```python
from build123d import *

# Parameters (mm, degrees)
SKETCH_1_R      = 12.5
EXTRUDE_1_DEPTH = 5
EXTRUDE_2_DEPTH = 5


with BuildPart() as part:
    # ｽｹｯﾁ1 → ﾎﾞｽ - 押し出し1 (new body)
    with BuildSketch(Plane.XY):
        with Locations((-14.880131723, 17.607142857)):
            Circle(SKETCH_1_R)
    extrude(amount=EXTRUDE_1_DEPTH)

    # ｽｹｯﾁ2 → ﾎﾞｽ - 押し出し2 (add)
    with BuildSketch(Plane(origin=(0, 0, 0), x_dir=(-1, 0, 0), z_dir=(0, 0, -1))):
        Polygon((13.880131723, 30.067078652), (16.678684785, 29.977074421), (18.364346975, 35.725860639), (16.86512212, 35.774077191), (14.066569059, 35.864081422), (12.567344204, 35.912297974), align=None)
    extrude(amount=-EXTRUDE_2_DEPTH)


solid = part.part
```
Input: part model. Units: mm. Frame: model coordinates. A direction names the side the tool comes from. Give positions to 0.01 mm unless a question says otherwise; leave off trailing zeros. Order: outer loops, then holes, each group sorted by start corner. A loop starts at its lowest first (then second) coordinate and runs counter-clockwise, first axis right, second up. Notation, with made-up numbers: M -39,-1.5 L -3,-1.5 A36 cw -3,36.5 Z; hole C 68.5,81.5 d5. An arc over 180 degrees is marked long. Return JSON: item names as keys, results as strings.
1) Section query C-C on x = -10. Output: boundary loops of the cut face in (y, z).
Taken from the geometry:
{"outline": "M 6.1,0 L 29.12,0 L 29.12,5 L 6.1,5 Z"}
2) Section query A-A on z = 1.85. Output: boundary loops of the cut face in (x, y), and give its area (3 significant figures).
Taken from the geometry:
{"outline": "M -18.36,35.73 L -16.68,29.98 A12.5 ccw long -13.88,30.07 L -12.57,35.91 Z", "area": "516 mm2"}
3) Line query: L1, parallel to X at y = 10.5, z = 3.85; L2, parallel to Y at x = -20.75, z = 3.7; L3, parallel to X at y = 7, z = 2. Output: solid intervals per line, ascending. Write a range as [from, to].
Taken from the geometry:
{"L1": "x = [-25.16, -4.6]", "L2": "y = [6.57, 28.64]", "L3": "x = [-21.49, -8.27]"}
4) Mould query, pull axis Y, two halves, no side actions, for faces 1 (the face through (-15, 17, 5)), 2 (the face through (-13.215, 33.031, 2.465)). Classes: released by +Y, released by -Y, zero draft, split by the parting line, or undercut.
Taken from the geometry:
{"face 1": "zero draft", "face 2": "undercut"}
5) Contact query for flat-ended pins moving along their axis: pin 1 (2 mm diameter, centred on y = 11.5, z = 2.5, fed in from -X); pin 2 (2 mm diameter, centred on x = -7, z = 0.5, fed in from +Y). Output: stop coordinate, or through.
Taken from the geometry:
{"pin 1": "stops at x = -26.29", "pin 2": "stops at y = 28.04"}
6) Section query B-B on y = 22. Output: boundary loops of the cut face in (x, z), and give its area (3 significant figures).
Taken from the geometry:
{"outline": "M -26.58,0 L -3.18,0 L -3.18,5 L -26.58,5 Z", "area": "117 mm2"}
7) Access query for faces 3 (the face through (-17.51, 32.81, 2.46)), 4 (the face through (-15.008, 5.108, 2.465)). Directions: +Z, -Z, +X, -X, +Y, -Y. A direction counts if a zero-diameter tool reaches every point of the face in a straight line with its end or side. Return the directions, or none.
Taken from the geometry:
{"face 3": "+Z, -Z, -X", "face 4": "+Z, -Z"}
